Here's how the part is built. I have some questions about the finished solid (model axes, mm). A direction names the side the tool comes from. Give positions to 0.01 mm unless a question says otherwise; leave off trailing zeros. Order: outer loops, then holes, each group sorted by start corner. A loop starts at its lowest first (then second) coordinate and runs counter-clockwise, first axis right, second up. Notation, with made-up numbers: (7, 19.25) - (64, 19.25) arc R6 ccw to (64, 29.25) - close; hole circle Ø9 at (-8, -23.5). An arc over 180 degrees is marked (long way). One line per question, with ' | ' between items.
Autodesk Fusion 360 part; units mm, degrees
sketch "Sketch1" plane through (0, 0, 0) normal (1, 0, 0) x (0, 0, -1)
  line L0 (-44.5, 28) -> (44.5, 28)
  line L1 (44.5, 28) -> (44.5, -28)
  line L2 (44.5, -28) -> (-44.5, -28)
  line L3 (-44.5, -28) -> (-44.5, 28)
  line L4 (-44.5, 28) -> (44.5, -28) construction
  line L5 (44.5, 28) -> (-44.5, -28) construction
  circle A0 centre (-38, 24.5) radius 1.25
  circle A1 centre (-38, -24.5) radius 1.25
  circle A2 centre (20, 25.1038) radius 1.25
  circle A3 centre (20, -23.8962) radius 1.25
  line L6 (-52, 35.5) -> (52, 35.5)
  line L7 (52, 35.5) -> (52, -35.5)
  line L8 (52, -35.5) -> (-52, -35.5)
  line L9 (-52, -35.5) -> (-52, 35.5)
  line L10 (-52, 35.5) -> (52, -35.5) construction
  line L11 (52, 35.5) -> (-52, -35.5) construction
  line L12 (-44.5, 28) -> (-44.5, 29)
  line L13 (-44.5, 29) -> (44.5, 29)
  line L14 (44.5, 29) -> (44.5, 28)
  circle A4 centre (0, 0) radius 13.5
  line L15 (-15, 15) -> (15, 15)
  line L16 (15, 15) -> (15, -15)
  line L17 (15, -15) -> (-15, -15)
  line L18 (-15, -15) -> (-15, 15)
  line L19 (-15, 15) -> (15, -15) construction
  line L20 (15, 15) -> (-15, -15) construction
  circle A5 centre (13, 13) radius 1.5
  circle A6 centre (-13, 13) radius 1.5
  circle A7 centre (-13, -13) radius 1.5
  circle A8 centre (13, -13) radius 1.5
  dimension "d1" = 89
  dimension "d2" = 56
  dimension "d3" = 2.5
  dimension "d4" = 3.5
  dimension "d5" = 6.5
  dimension "d6" = 2.5
  dimension "d7" = 6.5
  dimension "d8" = 49
  dimension "d9" = 2.5
  dimension "d10" = 2.5
  dimension "d11" = 49
  dimension "d12" = 58
  dimension "d13" = 58
  dimension "d16" = 104
  dimension "d17" = 71
  dimension "d86" = 27
  dimension "d87" = 30
  dimension "d88" = 30
  dimension "d89" = 3
  dimension "d90" = 3
  dimension "d91" = 3
  dimension "d92" = 3
  dimension "d93" = 2
  dimension "d94" = 2
  dimension "d95" = 2
  dimension "d96" = 2
extrude "Extrude1" add sketch "Sketch1" along normal blind 2 contours L0 L12 L13 L14 | L0 L1 L2 L3 | L15 L16 L17 L18
extrude "Extrude2" add sketch "Sketch1" along normal blind 50 contours L6 L7 L8 L9
sketch "Sketch2" plane through (0, -28, 0) normal (0, 1, 0) x (-1, 0, 0)
  line L0 (-2, -44.5) -> (-2, 44.5)
  line L1 (-2, 44.5) -> (-50, 44.5)
  line L2 (-50, 44.5) -> (-50, -44.5)
  line L3 (-50, -44.5) -> (-2, -44.5)
  line L4 (-9, 34.9) -> (-12, 34.9)
  line L5 (-12, 34.9) -> (-12, 26.9)
  line L6 (-12, 26.9) -> (-9, 26.9)
  line L7 (-9, 26.9) -> (-9, 34.9)
  line L8 (-12, 34.9) -> (-50, 34.9)
  line L9 (-50, 34.9) -> (-50, 26.9)
  line L10 (-50, 26.9) -> (-12, 26.9)
  line L11 (-12, 26.9) -> (-12, 34.9)
  line L12 (-9, 14.4989) -> (-9, 4.4989)
  line L13 (-9, 4.4989) -> (-11.002, 2)
  line L14 (-11.002, 2) -> (-15.002, 2)
  line L15 (-15.002, 2) -> (-15.002, 17)
  line L16 (-15.002, 17) -> (-11.002, 17)
  line L17 (-11.002, 17) -> (-9, 14.4989)
  line L18 (-15.002, 17) -> (-50, 17)
  line L19 (-50, 17) -> (-50, 2)
  line L20 (-50, 2) -> (-15.002, 2)
  line L21 (-15.002, 2) -> (-15.002, 17)
  line L22 (-9, -8.5) -> (-16, -8.5)
  line L23 (-16, -8.5) -> (-16, -15.5)
  line L24 (-16, -15.5) -> (-9, -15.5)
  line L25 (-9, -15.5) -> (-9, -8.5)
  line L26 (-16, -8.5) -> (-50.0121, -8.5)
  line L27 (-50.0121, -8.5) -> (-50.0121, -15.5)
  line L28 (-50.0121, -15.5) -> (-16, -15.5)
  line L29 (-16, -15.5) -> (-16, -8.5)
  dimension "d20" = 3
  dimension "d21" = 8
  dimension "d22" = 9.6
  dimension "d30" = 10
  dimension "d33" = 4
  dimension "d34" = 15
  dimension "d35" = 4
  dimension "d36" = 7
  dimension "d37" = 7
  dimension "d38" = 27.5
  dimension "d39" = 7
  dimension "d40" = 7
  dimension "d41" = 7
  dimension "d42" = 53
extrude "Extrude3" cut sketch "Sketch2" against normal blind 2.5 contours L2 L26 L27 L28 | L2 L23 L26 L28 L29 | L2 L5 L8 L9 L10 L11 | L22 L23 L24 L25 L29 | L4 L5 L6 L7 L11 | L2 L15 L18 L19 L20 L21 | L12 L13 L14 L15 L16 L17 L21
sketch "Sketch3" plane through (0, -35.5, 0) normal (0, -1, 0) x (1, 0, 0)
  line L0 (0, 52) -> (0, -52)
  line L1 (0, -52) -> (50, -52)
  line L2 (50, -52) -> (50, 52)
  line L3 (50, 52) -> (0, 52)
  line L4 (19.5, 21) -> (4.5, 21)
  line L5 (4.5, 21) -> (4.5, -2)
  line L6 (4.5, -2) -> (19.5, -2)
  line L7 (19.5, -2) -> (19.5, 21)
  line L8 (19.5, 21) -> (50, 21)
  line L9 (50, 21) -> (50, -2)
  line L10 (50, -2) -> (19.5, -2)
  line L11 (19.5, -2) -> (19.5, 21)
  dimension "d45" = 15
  dimension "d46" = 23
  dimension "d47" = 31
  dimension "d48" = 4.5
extrude "Extrude4" cut sketch "Sketch3" against normal blind 5.5 contours L2 L7 L8 L9 L10 L11 | L4 L5 L6 L7 L11
sketch "Sketch4" plane through (0, 0, -44.5) normal (0, 0, 1) x (1, 0, 0)
  line L0 (2, 29) -> (2, -28)
  line L1 (2, -28) -> (50, -28)
  line L2 (50, -28) -> (50, 29)
  line L3 (9, -25.75) -> (22.5, -25.75)
  line L4 (22.5, -25.75) -> (22.5, -9.75)
  line L5 (22.5, -9.75) -> (9, -9.75)
  line L6 (9, -9.75) -> (9, -25.75)
  line L7 (25, -6.5) -> (9, -6.5)
  line L8 (9, -6.5) -> (9, 8.5)
  line L9 (9, 8.5) -> (25, 8.5)
  line L10 (25, 8.5) -> (25, -6.5)
  line L11 (25, 11.5) -> (9, 11.5)
  line L12 (9, 11.5) -> (9, 26.5)
  line L13 (9, 26.5) -> (25, 26.5)
  line L14 (25, 26.5) -> (25, 11.5)
  line L15 (25, 26.5) -> (50, 26.5)
  line L16 (50, 26.5) -> (50, 11.5)
  line L17 (50, 11.5) -> (25, 11.5)
  line L18 (25, 11.5) -> (25, 26.5)
  line L19 (25, 8.5) -> (50, 8.5)
  line L20 (50, 8.5) -> (50, -6.5)
  line L21 (50, -6.5) -> (25, -6.5)
  line L22 (25, -6.5) -> (25, 8.5)
  line L23 (22.5, -9.75) -> (50, -9.75)
  line L24 (50, -9.75) -> (50, -25.75)
  line L25 (50, -25.75) -> (22.5, -25.75)
  line L26 (22.5, -25.75) -> (22.5, -9.75)
  line L27 (50, 29) -> (2, 29)
  dimension "d51" = 13.5
  dimension "d52" = 16
  dimension "d53" = 2.25
  dimension "d54" = 7
  dimension "d55" = 16
  dimension "d56" = 15
  dimension "d57" = 7
  dimension "d58" = 21.5
  dimension "d59" = 16
  dimension "d60" = 15
  dimension "d61" = 7
  dimension "d62" = 39.5
  dimension "d65" = 15
extrude "Extrude5" cut sketch "Sketch4" against normal blind 3 contours L2 L14 L15 L16 L17 L18 | L2 L4 L23 L24 L25 L26 | L11 L12 L13 L14 L18 | L3 L4 L5 L6 L26 | L2 L10 L19 L20 L21 L22 | L7 L8 L9 L10 L22
sketch "Sketch5" plane through (0, 0, -52) normal (0, 0, -1) x (-1, 0, 0)
  line L0 (0, -35.5) -> (0, 35.5)
  line L1 (0, 35.5) -> (-50, 35.5)
  line L2 (-50, 35.5) -> (-50, -35.5)
  line L3 (-50, -35.5) -> (0, -35.5)
  line L4 (-7, -26.75) -> (-23, -26.75)
  line L5 (-23, -26.75) -> (-23, -8.75)
  line L6 (-23, -8.75) -> (-7, -8.75)
  line L7 (-7, -8.75) -> (-7, -26.75)
  line L8 (-23, -8.75) -> (-50, -8.75)
  line L9 (-50, -8.75) -> (-50, -26.75)
  line L10 (-50, -26.75) -> (-23, -26.75)
  line L11 (-23, -26.75) -> (-23, -8.75)
  dimension "d66" = 16
  dimension "d67" = 18
  dimension "d68" = 8.75
  dimension "d69" = 7
extrude "Extrude6" cut sketch "Sketch5" against normal blind 4.5 contours L2 L5 L8 L9 L10 L11 | L4 L5 L6 L7 L11
sketch "Sketch6" plane through (50, 0, 0) normal (1, 0, 0) x (0, 0, -1)
  line L0 (47.5, -8.75) -> (52, -8.75)
  line L1 (52, -8.75) -> (52, 35.5)
  line L2 (52, 35.5) -> (-52, 35.5)
  line L3 (-52, 35.5) -> (-52, -35.5)
  line L4 (-52, -35.5) -> (-21, -35.5)
  line L5 (-21, -35.5) -> (-21, -30)
  line L6 (-21, -30) -> (-17, -30)
  line L7 (-17, -30) -> (-17, -28)
  line L8 (-17, -28) -> (-26.9, -28)
  line L9 (-26.9, -28) -> (-26.9, -30.5)
  line L10 (-26.9, -30.5) -> (-34.9, -30.5)
  line L11 (-34.9, -30.5) -> (-34.9, -28)
  line L12 (-34.9, -28) -> (-44.5, -28)
  line L13 (-44.5, -28) -> (-44.5, 29)
  line L14 (44.5, 29) -> (44.5, 26.5)
  line L15 (44.5, 26.5) -> (47.5, 26.5)
  line L16 (47.5, 26.5) -> (47.5, 11.5)
  line L17 (47.5, 11.5) -> (44.5, 11.5)
  line L18 (44.5, 11.5) -> (44.5, 8.5)
  line L19 (44.5, 8.5) -> (47.5, 8.5)
  line L20 (47.5, 8.5) -> (47.5, -6.5)
  line L21 (47.5, -6.5) -> (44.5, -6.5)
  line L22 (44.5, -6.5) -> (44.5, -9.75)
  line L23 (44.5, -9.75) -> (47.5, -9.75)
  line L24 (47.5, -9.75) -> (47.5, -8.75)
  circle A0 centre (-47.75, 31.25) radius 2
  circle A1 centre (-47.75, -31.25) radius 2
  circle A2 centre (47.75, 31.25) radius 2
  circle A3 centre (47.75, -31.25) radius 2
  line L25 (52, -35.5) -> (52, -26.75)
  line L26 (2, -35.5) -> (52, -35.5)
  line L27 (-44.5, 29) -> (44.5, 29)
  dimension "d72" = 4
  dimension "d73" = 4
  dimension "d74" = 4
  dimension "d75" = 4
  dimension "d76" = 4.25
  dimension "d77" = 4.25
  dimension "d78" = 4.25
  dimension "d79" = 4.25
  dimension "d80" = 4.25
  dimension "d81" = 4.25
  dimension "d82" = 4.25
  dimension "d83" = 4.25
extrude "Extrude7" cut sketch "Sketch6" against normal blind 4.75 contours A0 | A1 | A2 | A3
1) I want a section at D-D (z = -36). List the corners of the cut face in (x, y) for me, plus the area to 3 significant figures.
Model answer:
outline: (0, -35.5) - (50, -35.5) - (50, -28) - (2, -28) - (2, 29) - (50, 29) - (50, 35.5) - (0, 35.5) - close | area: 814 mm2
2) Please list where these lines run through material, in increasing order: L1, parallel to Y at x = 39, z = -47; L2, parallel to Y at x = 0.6, z = 38; L3, parallel to Y at x = 25.5, z = 40.
Model answer:
L1: y = -35.5 to -25.75, -9.75 to -6.5, 8.5 to 11.5, 26.5 to 35.5 | L2: y = -35.5 to -25.75, -23.25 to 23.25, 25.75 to 35.5 | L3: y = -35.5 to -28, 29 to 35.5
3) I want a section at B-B (z = -20). List the corners of the cut face in (x, y) for me, plus the area to 3 significant figures.
Model answer:
outline: (0, -35.5) - (50, -35.5) - (50, -28) - (2, -28) - (2, -25.15) - (0, -25.15) - close; (0, -22.65) - (2, -22.65) - (2, 23.85) - (0, 23.85) - close; (0, 26.35) - (2, 26.35) - (2, 29) - (50, 29) - (50, 35.5) - (0, 35.5) - close | area: 804 mm2
4) On a 3-axis mill with a long thin cutter (end or side, diameter ignored), from which of +Z, -Z, +X, -X, +Y, -Y can I reach the whole of each face in a straight line? I mean faces 1 (the face through (0.99, -13.07, -11.5)), 2 (the face through (30, -29, -15.5)), 3 (the face through (28, -8.75, -50)). Say none if no direction works.
Model answer:
face 1: +X, -X | face 2: +X | face 3: -Z, +X
5) I want a section at C-C (y = -18). List the corners of the cut face in (x, z) for me, plus the area to 4 significant figures.
Model answer:
outline: (0, -52) - (7, -52) - (7, -47.5) - (9, -47.5) - (9, -44.5) - (2, -44.5) - (2, 44.5) - (50, 44.5) - (50, 52) - (0, 52) - close | area: 611.5 mm2
6) I'm going to push flat-ended pins straight in: P1, Ø1.2, axis at y = 31.5, z = 47, coming from the +X side; P2, Ø4, axis at y = 13, z = -13, coming from the +X side; P3, Ø2, axis at y = -29, z = 8.5, coming from the +X side. Where does each tip first touch, or does it pass through?
Model answer:
P1: stops at x = 45.25 | P2: stops at x = 2 | P3: stops at x = 9
7) I want a section at A-A (y = 0). List the corners of the cut face in (x, z) for me.
Model answer:
outline: (0, -52) - (50, -52) - (50, -47.5) - (9, -47.5) - (9, -44.5) - (2, -44.5) - (2, -13.5) - (0, -13.5) - close; (0, 13.5) - (2, 13.5) - (2, 44.5) - (50, 44.5) - (50, 52) - (0, 52) - close
8) Thinking about a two-plate mould opening in Y: for faces 4 (the face through (25, 35.5, 1)), 5 (the face through (30, -29, 26.9)), 6 (the face through (25, 0, 52)), which applies, +Y half, -Y half, draft (parallel to the pull), parting line (faces both ways), or undercut?
Model answer:
face 4: +Y half | face 5: undercut | face 6: draft
